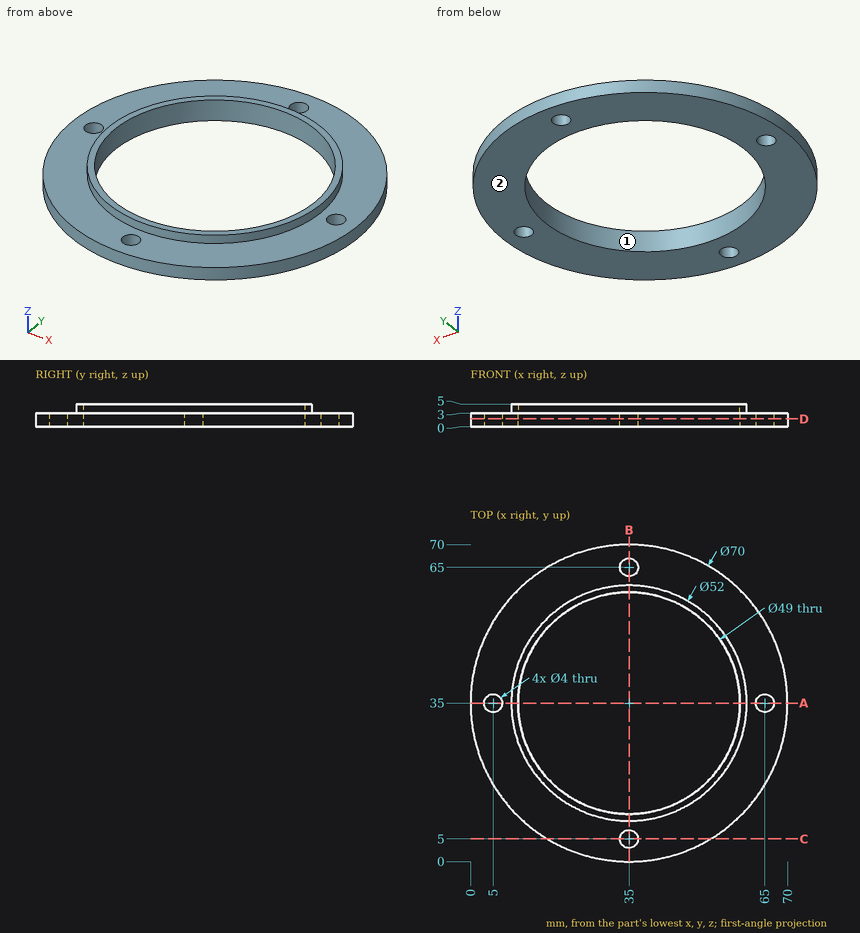
Could you check a few things on this drawing? It's one solid part, dimensions in mm from its lowest x, y, z. Coordinates: 2 decimals unless noted, no trailing zeros. Write each loop counter-clockwise with the first axis right and the second up, starting at its lowest first coordinate (ties: lowest second). Pieces come first, ordered by that corner, then holes.
1) Thinking about a two-plate mould opening in X: for the marked faces 1 and 2, which applies, +X half, -X half, draft (parallel to the pull), parting line (faces both ways), or undercut?
Filled in:
face 1: undercut
face 2: draft
2) If we section it at D-D (z = 1.7): List the corners of the cut face in (x, y) for me, plus the area to 3 significant figures.
Filled in:
outline: circle Ø70 at (35, 35); hole circle Ø4 at (5, 35); hole circle Ø49 at (35, 35); hole circle Ø4 at (35, 5); hole circle Ø4 at (35, 65); hole circle Ø4 at (65, 35)
area: 1,910 mm2
3) If we section it at C-C (y = 5): List the corners of the cut face in (x, z) for me.
Filled in:
outline: (16.97, 0) - (33, 0) - (33, 3) - (16.97, 3) - close; (37, 0) - (53.03, 0) - (53.03, 3) - (37, 3) - close
4) If I drill on line 1 (Y direction, x = 35, z = 1.8); line 2 (Y direction, x = 35, z = 3.55); line 3 (X direction, y = 33.5, z = 2.9), over which ranges is the centre line in solid material (lowest first)?
Filled in:
line 1: y = 0 to 3, 7 to 10.5, 59.5 to 63, 67 to 70
line 2: y = 9 to 10.5, 59.5 to 61
line 3: x = 0.03 to 3.68, 6.32 to 10.55, 59.45 to 63.68, 66.32 to 69.97
5) I'm going to push flat-ended pins straight in: pin 1 (1.5 mm diameter, centred on x = 16, z = 3.5, fed in from +Y); pin 2 (5 mm diameter, centred on x = 35, y = 5, fed in from +Z); pin 3 (3 mm diameter, centred on x = 45.5, z = 2, fed in from -Y). Where does each tip first touch, or does it pass through?
Filled in:
pin 1: stops at y = 64.75
pin 2: stops at z = 3
pin 3: stops at y = 1.18
6) If we section it at A-A (y = 35): List the corners of the cut face in (x, z) for me.
Filled in:
outline: (0, 0) - (3, 0) - (3, 3) - (0, 3) - close; (7, 0) - (10.5, 0) - (10.5, 5) - (9, 5) - (9, 3) - (7, 3) - close; (59.5, 0) - (63, 0) - (63, 3) - (61, 3) - (61, 5) - (59.5, 5) - close; (67, 0) - (70, 0) - (70, 3) - (67, 3) - close
